The listing builds one solid part. Answer for the finished solid, in the listing's coordinates (mm). A direction names the side the tool comes from. Give positions to 0.01 mm unless a question says otherwise; leave off trailing zeros. Loops run counter-clockwise (first coordinate to the right, second up) from the corner with the lowest first, then second, coordinate; pieces in that order, holes last.
Item 1: Section C-C, the plane z = 2.05 is taken. Give the number of separate pieces and of enclosed holes in the cut face, and give its area (3 significant figures).
Item 2: Section A-A, the plane x = 57.15 is taken. Give the vertices of the cut face in (y, z).
Item 3: Consider line 1 along Y through (x, z) = (165.1, 2.7); line 2 along Y through (x, z) = (192, 1.6); line 3 along X through (y, z) = (21.5, 2.15). Determine where each line is inside the solid, lowest interval first.
Item 4: Section B-B, the plane y = 50.8 is taken. Give the vertices of the cut face in (x, z), and give its area (3 significant figures).
Item 5: A tool of negligible diameter and unlimited length cuts with its end or side. For faces 4 (the face through (167.37, 102.32, 2.41)), 5 (the face through (152.4, 6, 2)), 6 (the face through (25.4, 19, 2)), from which of +Z, -Z, +X, -X, +Y, -Y can it reach the whole face along a straight path? Write none if from no direction.
Item 6: Section D-D, the plane x = 165.1 is taken. Give the vertices of the cut face in (y, z), and give its area (3 significant figures).
Item 7: Each of these flat-tipped pins is pushed along its axis until it touches: pin 1 Ø5.5 at (x, y) = (165.1, 101.6) entering from +Z; pin 2 Ø1 at (x, z) = (132.5, 2) entering from +Y; pin 3 Ø2.5 at (x, z) = (15, 2) entering from -Y; pin 4 Ø1.4 at (x, z) = (168, 2) entering from -Y. Where does it stop, or does it pass through?
Item 8: The mould has two halves that part along Y. Classify faces 1 (the face through (167.37, 51.52, 2.41)), 2 (the face through (78.09, 89.53, 2.41)), 3 (the face through (203.2, 63, 2)): pulls with the +Y half, pulls with the -Y half, needs draft (parallel to the pull), parting line crosses it, or undercut.
Autodesk Inventor part; units mm, degrees
ref_plane "YZ Plane" through (0, 0, 0) normal (1, 0, 0) x (0, 1, 0)
ref_plane "XZ Plane" through (0, 0, 0) normal (0, 1, 0) x (-1, 0, 0)
ref_plane "XY Plane" through (0, 0, 0) normal (0, 0, 1) x (1, 0, 0)
sketch "Sketch1" plane through (0, 0, 0) normal (0, 0, 1) x (1, 0, 0)
  line L0 (0, 0) -> (203.2, 0)
  line L1 (203.2, 0) -> (203.2, 127)
  line L2 (203.2, 127) -> (0, 127)
  line L3 (0, 127) -> (0, 0)
  dimension "d0" = 203.2
  dimension "d1" = 127
extrude "Extrusion1" add sketch "Sketch1" along normal blind 4.7625
sketch "Sketch2" plane through (0, 0, 4.7625) normal (0, 0, 1) x (1, 0, 0)
  line L0 (203.2, 127) -> (203.2, 0)
  line L1 (0, 127) -> (203.2, 127)
  line L2 (190.5, 127) -> (190.5, 101.6) construction
  circle A0 centre (190.5, 101.6) radius 2.3813
  dimension "d4" = 4.7625
  dimension "d5" = 25.4
  dimension "d6" = 12.7
extrude "Extrusion2" cut sketch "Sketch2" against normal up to next
pattern_linear "Rectangular Pattern1" count 4 spacing 25.4 along (0, -1, 0) count 2 spacing 25.4 along (-1, 0, 0) of "Extrusion2"
sketch "Sketch3" plane through (0, 0, 4.7625) normal (0, 0, 1) x (1, 0, 0)
  line L0 (203.2, 0) -> (0, 0)
  line L1 (203.2, 127) -> (203.2, 0)
  circle A0 centre (114.3, 12.7) radius 4.7625
  circle A1 centre (57.15, 38.1) radius 4.7625
  dimension "d15" = 9.525
  dimension "d16" = 88.9
  dimension "d17" = 12.7
  dimension "d18" = 57.15
  dimension "d19" = 25.4
extrude "Extrusion3" cut sketch "Sketch3" against normal up to next
sketch "Sketch4" plane through (0, 0, 4.7625) normal (0, 0, 1) x (1, 0, 0)
  line L0 (0, 0) -> (0, 127)
  line L1 (0, 0) -> (25.4, 0)
  line L2 (25.4, 0) -> (25.4, 38.1)
  line L3 (25.4, 38.1) -> (0, 38.1)
  line L4 (0, 38.1) -> (0, 0)
  line L5 (203.2, 127) -> (0, 127)
  line L6 (0, 127) -> (0, 114.3)
  line L7 (0, 114.3) -> (203.2, 114.3)
  line L8 (203.2, 114.3) -> (203.2, 127)
  line L9 (203.2, 0) -> (152.4, 0)
  line L10 (152.4, 0) -> (152.4, 12.7)
  line L11 (152.4, 12.7) -> (203.2, 12.7)
  line L12 (203.2, 12.7) -> (203.2, 0)
  dimension "d22" = 38.1
  dimension "d23" = 25.4
  dimension "d24" = 50.8
  dimension "d25" = 12.7
  dimension "d26" = 12.7
extrude "Extrusion4" cut sketch "Sketch4" against normal up to next
sketch "Sketch5" plane through (0, 0, 4.7625) normal (0, 0, 1) x (1, 0, 0)
  line L0 (203.2, 114.3) -> (0, 114.3)
  line L1 (0, 38.1) -> (0, 114.3)
  line L2 (0, 114.3) -> (0, 63.5)
  line L3 (152.4, 114.3) -> (0, 63.5)
  line L4 (0, 114.3) -> (152.4, 114.3)
  point P0 (0, 0)
  dimension "d29" = 25.4
  dimension "d30" = 50.8
extrude "Extrusion5" cut sketch "Sketch5" against normal up to next
fillet "Fillet1" radius 3.175 9 edges at (0, 63.5, 2.3813) (0, 38.1, 2.3813) (25.4, 0, 2.3813) (152.4, 114.3, 2.3813) (203.2, 114.3, 2.3813) (203.2, 12.7, 2.3813) (152.4, 12.7, 2.3813) (152.4, 0, 2.3813) (25.4, 38.1, 2.3813)
properties part number "Frame_BottomRollerPlate" material "Aluminum-6061"
Worked answers:
1. separate pieces: 1
1. enclosed holes: 10
1. area: 17,400 mm2
2. outline: (0, 0) - (33.34, 0) - (33.34, 4.76) - (0, 4.76) - close; (42.86, 0) - (82.55, 0) - (82.55, 4.76) - (42.86, 4.76) - close
3. line 1: y = 12.7 to 23.02, 27.78 to 48.42, 53.18 to 73.82, 78.58 to 99.22, 103.98 to 114.3
3. line 2: y = 12.7 to 23.55, 27.25 to 48.95, 52.65 to 74.35, 78.05 to 99.75, 103.45 to 114.3
3. line 3: x = 25.4 to 203.2
4. outline: (0, 0) - (162.72, 0) - (162.72, 4.76) - (0, 4.76) - close; (167.48, 0) - (188.12, 0) - (188.12, 4.76) - (167.48, 4.76) - close; (192.88, 0) - (203.2, 0) - (203.2, 4.76) - (192.88, 4.76) - close
4. area: 922 mm2
5. face 4: +Z, -Z
5. face 5: +Z, -Z, +X, -Y
5. face 6: +Z, -Z, -X, -Y
6. outline: (12.7, 0) - (23.02, 0) - (23.02, 4.76) - (12.7, 4.76) - close; (27.78, 0) - (48.42, 0) - (48.42, 4.76) - (27.78, 4.76) - close; (53.18, 0) - (73.82, 0) - (73.82, 4.76) - (53.18, 4.76) - close; (78.58, 0) - (99.22, 0) - (99.22, 4.76) - (78.58, 4.76) - close; (103.98, 0) - (114.3, 0) - (114.3, 4.76) - (103.98, 4.76) - close
6. area: 393 mm2
7. pin 1: stops at z = 4.76
7. pin 2: stops at y = 107.83
7. pin 3: stops at y = 38.1
7. pin 4: stops at y = 12.7
8. face 1: undercut
8. face 2: pulls with the +Y half
8. face 3: needs draft
